Verification items for the finished model (mm, model axes). Face numbers are marked on the shaded views. A direction names the side the tool comes from. Coordinates: 2 decimals unless noted, no trailing zeros. Write each loop counter-clockwise with the first axis right and the second up, starting at its lowest first coordinate (ties: lowest second). Pieces come first, ordered by that corner, then holes. Notation, with made-up numbers: M 35.5,57.5 L 57.5,57.5 A18 cw 57.5,63.5 Z; hole C 1,-38 d7. An arc over 180 degrees is marked long. Answer in a Markdown table with one row per item.
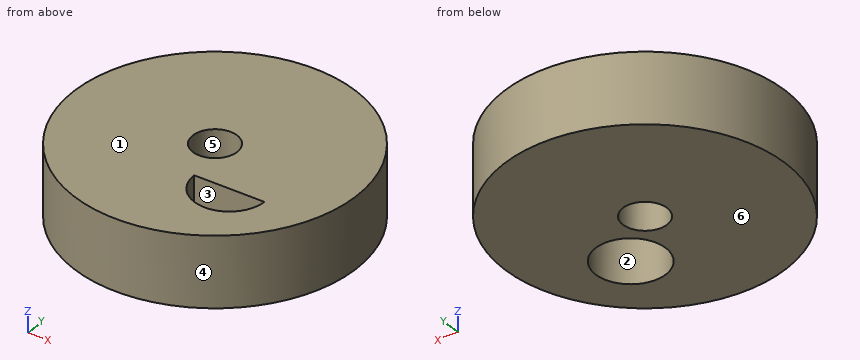
from build123d import *

# Parameters (mm, degrees)
SKETCH1_R           = 25.4
SKETCH1_R_2         = 4.0000047
BOSS_EXTRUDE1_DEPTH = 12.7
SKETCH2_R           = 6.35
CUT_EXTRUDE1_DEPTH  = 6.35
CUT_EXTRUDE2_DEPTH  = 12.7


with BuildPart() as part:
    # Sketch1 → Boss-Extrude1 (new body)
    with BuildSketch(Plane.XY):
        Circle(SKETCH1_R)
        Circle(SKETCH1_R_2, mode=Mode.SUBTRACT)
    extrude(amount=BOSS_EXTRUDE1_DEPTH)

    # Sketch2 → Cut-Extrude1 (cut)
    with BuildSketch(Plane.XY):
        with Locations((8.89, -8.89)):
            Circle(SKETCH2_R)
    extrude(amount=CUT_EXTRUDE1_DEPTH, mode=Mode.SUBTRACT)

    # Sketch3 → Cut-Extrude2 (cut)
    with BuildSketch(Plane.XY):
        with BuildLine():
            Line((2.54, -8.89), (15.24, -8.89))
            ThreePointArc((15.24, -8.89), (8.89, -15.24), (2.54, -8.89))
        make_face()
    extrude(amount=CUT_EXTRUDE2_DEPTH, mode=Mode.SUBTRACT)


solid = part.part
1) Thickness scan on L1, parallel to Y at x = 0, z = 1.25; L2, parallel to Y at x = 5, z = 2; L3, parallel to X at y = -6.5, z = 2. Record the ranges inside material, lowest first. Write a range as [from, to].
Response values:
| item | result |
|---|---|
| L1 | y = [-25.4, -4], [4, 25.4] |
| L2 | y = [-24.9, -13.91], [-3.87, 24.9] |
| L3 | x = [-24.55, 3.01], [14.77, 24.55] |
2) Sectioned sample at D-D (x = 8.89). Record the cut outline in (y, z).
Response values:
| item | result |
|---|---|
| outline | M -23.79,0 L -15.24,0 L -15.24,12.7 L -23.79,12.7 Z; M -8.89,6.35 L -2.54,6.35 L -2.54,0 L 23.79,0 L 23.79,12.7 L -8.89,12.7 Z |
3) Depth check by flat-ended pin: pin 1 (3 mm diameter, centred on x = 9, z = 2, fed in from +Y); pin 2 (6 mm diameter, centred on y = -11.5, z = 4, fed in from +X); pin 3 (2 mm diameter, centred on x = 10, z = 5.5, fed in from +Y); pin 4 (7 mm diameter, centred on x = 0, y = 0, fed in from +Z). Enter the tip coordinate at first touch or a pass-through.
Response values:
| item | result |
|---|---|
| pin 1 | stops at y = 24.27 |
| pin 2 | stops at x = 23.94 |
| pin 3 | stops at y = 23.75 |
| pin 4 | passes through |
4) Sectioned sample at A-A (x = 0). Record the cut outline in (y, z), then the cut area to 3 significant figures.
Response values:
| item | result |
|---|---|
| outline | M -25.4,0 L -4,0 L -4,12.7 L -25.4,12.7 Z; M 4,0 L 25.4,0 L 25.4,12.7 L 4,12.7 Z |
| area | 544 mm² |
5) Tool access check on the marked faces 1, 2 and 3. Record the directions out of +Z, -Z, +X, -X, +Y, -Y that give a thin tool (end or side, any length) a straight path to the whole face; none if there is none.
Response values:
| item | result |
|---|---|
| face 1 | +Z, +X, -X, +Y, -Y |
| face 2 | -Z |
| face 3 | +Z, -Z |
6) Sectioned sample at C-C (z = 3.75). Record the cut outline in (x, y).
Response values:
| item | result |
|---|---|
| outline | C 0,0 d50.8; hole C 0,0 d8; hole C 8.89,-8.89 d12.7 |
7) Release check for a two-part mould opening along X. For the marked faces 4, 5 and 6 record: +X half, -X half, draft (parallel to the pull), parting line (faces both ways), or undercut.
Response values:
| item | result |
|---|---|
| face 4 | parting line |
| face 5 | undercut |
| face 6 | draft |
